Part print with two shaded views. Sizes in mm from the minimum x, y, z corner. A direction names the side the tool comes from. Give positions to 0.01 mm unless a question says otherwise; leave off trailing zeros. Loops run counter-clockwise (first coordinate to the right, second up) from the corner with the lowest first, then second, coordinate; pieces in that order, holes last. Notation, with made-up numbers: M -37,29 L -28,29 A8 cw -28,34 Z; hole C 53.25,-30 d6. An arc over 180 degrees is marked long. Answer in a Markdown table with one row per item.
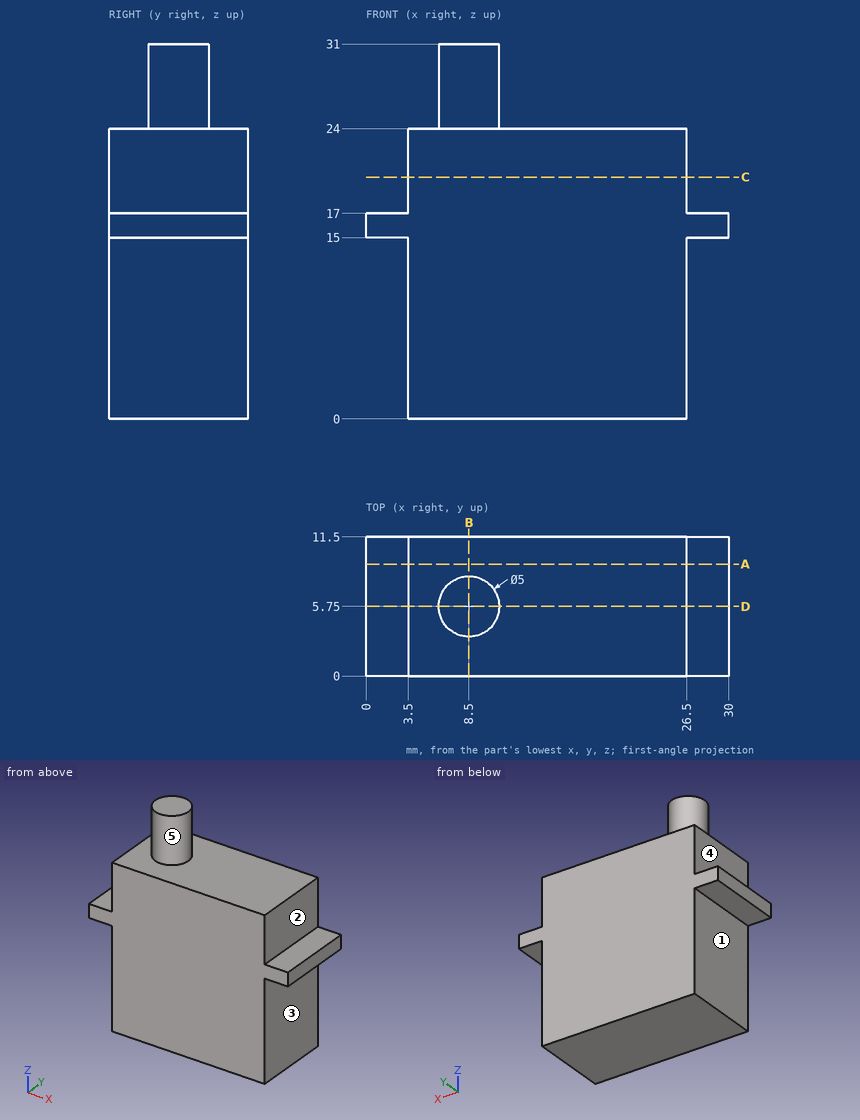
Q1. 3-axis set-ups, long thin cutter, end or side, ignore diameter. For the marked faces 1, 2, 3, 4 and 5: which of +Z, -Z, +X, -X, +Y, -Y reach the whole face in a straight line?
Reported:
| item | result |
|---|---|
| face 1 | -Z, -X, +Y, -Y |
| face 2 | +Z, +X, +Y, -Y |
| face 3 | -Z, +X, +Y, -Y |
| face 4 | +Z, -X, +Y, -Y |
| face 5 | +Z |
Q2. Saw through at C-C (z = 20). Give the cut face in (x, y), and give its area (4 significant figures).
Reported:
| item | result |
|---|---|
| outline | M 3.5,0 L 26.5,0 L 26.5,11.5 L 3.5,11.5 Z |
| area | 264.5 mm² |
Q3. Saw through at A-A (y = 9.25). Give the cut face in (x, z), and give its area (3 significant figures).
Reported:
| item | result |
|---|---|
| outline | M 0,15 L 3.5,15 L 3.5,0 L 26.5,0 L 26.5,15 L 30,15 L 30,17 L 26.5,17 L 26.5,24 L 3.5,24 L 3.5,17 L 0,17 Z |
| area | 566 mm² |
Q4. Saw through at D-D (y = 5.75). Give the cut face in (x, z).
Reported:
| item | result |
|---|---|
| outline | M 0,15 L 3.5,15 L 3.5,0 L 26.5,0 L 26.5,15 L 30,15 L 30,17 L 26.5,17 L 26.5,24 L 11,24 L 11,31 L 6,31 L 6,24 L 3.5,24 L 3.5,17 L 0,17 Z |
Q5. Drop flat-ended pins along their axis: pin 1 (1 mm diameter, centred on x = 27.5, y = 7, fed in from -Z); pin 2 (3.5 mm diameter, centred on y = 3.5, z = 20.5, fed in from +X); pin 3 (1 mm diameter, centred on x = 29, y = 4.5, fed in from +Z). Give the stop position or say it passes through.
Reported:
| item | result |
|---|---|
| pin 1 | z = 15 |
| pin 2 | x = 26.5 |
| pin 3 | z = 17 |
Q6. Saw through at B-B (x = 8.5). Give the cut face in (y, z), and give its area (3 significant figures).
Reported:
| item | result |
|---|---|
| outline | M 0,0 L 11.5,0 L 11.5,24 L 8.25,24 L 8.25,31 L 3.25,31 L 3.25,24 L 0,24 Z |
| area | 311 mm² |
Q7. Probe probe 1 along X at (y, z) = (10.75, 3); probe 2 along Z at (x, y) = (12.25, 3.25); probe 3 along Z at (x, y) = (28.25, 1). List the from-to ranges inside material, lowest first.
Reported:
| item | result |
|---|---|
| probe 1 | 3.5 to 26.5 |
| probe 2 | 0 to 24 |
| probe 3 | 15 to 17 |
